Geometry: final body of the model. Coordinates: model frame, mm. A direction names the side the tool comes from. Coordinates: 2 decimals unless noted, no trailing zeros. Order: outer loops, then holes, each group sorted by start corner. A loop starts at its lowest first (then second) coordinate and runs counter-clockwise, first axis right, second up. Notation, with made-up numbers: M 37.5,-14 L 55.5,-14 A11 ccw 55.5,3 Z; hole C -14.75,-17.5 d8. An arc over 180 degrees is marked long. Use CSV: the item, a comma, the result in double quotes. Start each with the question number.
1. Pull-direction query (Y, two-part tool) for faces 1 (the cylindrical face through (7.395, -1.494, 6.294)), 2 (the flat face through (0, -6, 0)), 3 (the cylindrical face through (7.4, 6.03, -2.24)); classes: pulls with the +Y half, pulls with the -Y half, needs draft (parallel to the pull), parting line crosses it, or undercut.
2. Material intervals for line 1 (Y direction, x = 5.5, z = 0); line 2 (Y direction, x = -2.5, z = 0); line 3 (Y direction, x = 8, z = 5.5), sorted ascending.
3. First-contact query: P1, Ø5, axis at x = 1.5, y = -2.5, coming from the -Z side; P2, Ø1.1, axis at y = 4.5, z = 4.5, coming from the -X side; P3, Ø1, axis at x = -1.5, y = -3, coming from the +Z side. Flat tips, straight axial feed; report the tip coordinate or a pass-through.
4. Section query A-A on x = -3. Return the cut outline in (y, z).
5. Set-up query: faces 4 (the flat face through (-10, -1, 0)), 5 (the flat face through (0, -3, -5)). Return all of +Z, -Z, +X, -X, +Y, -Y with unobstructed straight access to the full face (end or side cutting, diameter ignored); none if empty.
from build123d import *
from build123d.topology import SkipClean

# Parameters (mm, degrees)
BASPROSKE_W      = 15
BASPROSKE_H      = 7.5
TOOTHCUT_DEPTH   = 19.371173071
TEETHCUTS_COUNT  = 13
TEETHCUTS_ANGLE  = 332.307692308
HUBNEAONESKE_R   = 5.249
HUBNEARONE_DEPTH = 10.0000508
BORSKE_R         = 0.4
BORE_DEPTH       = 25.0000508


with BuildPart() as part:
    # BasProSke → Base-Revolve (revolve)
    with BuildSketch(Plane(origin=(0, 0, 0), x_dir=(1, 0, 0), z_dir=(0, 1, 0)), mode=Mode.PRIVATE) as base_revolve_sk:
        with Locations((7.5, 3.75)):
            Rectangle(BASPROSKE_W, BASPROSKE_H)
    revolve(base_revolve_sk.sketch.rotate(Axis((-10, 0, 0), (1, 0, 0)), 180), axis=Axis((-10, 0, 0), (1, 0, 0)))

    # TooCutSke → ToothCut (cut, through all)
    with BuildSketch(Plane(origin=(0, 0, 0), x_dir=(0, 0, -1), z_dir=(1, 0, 0))):
        with BuildLine():
            ThreePointArc((0.550489643, 5.220053846), (0, 5.249), (-0.550489643, 5.220053846))
            ThreePointArc((-0.550489643, 5.220053846), (-0.834571714, 6.414617604), (-1.635166801, 7.345602405))
            ThreePointArc((-1.635166801, 7.345602405), (0, 7.5254), (1.635166801, 7.345602405))
            ThreePointArc((1.635166801, 7.345602405), (0.834571714, 6.414617604), (0.550489643, 5.220053846))
        make_face()
    toothcut = extrude(amount=TOOTHCUT_DEPTH, mode=Mode.SUBTRACT)

    # TeethCuts: ToothCut ×13 about axis
    teethcuts_axis = Axis((-10, 0, 0), (1, 0, 0))
    for i in range(1, TEETHCUTS_COUNT):
        add(toothcut.rotate(teethcuts_axis, i * TEETHCUTS_ANGLE / (TEETHCUTS_COUNT - 1)), mode=Mode.SUBTRACT)

    # HubNeaOneSke → HubNearOne (add)
    with SkipClean():  # the faces are left unmerged after this step: merging them gives an invalid solid
        with BuildSketch(Plane.ZY):
            Circle(HUBNEAONESKE_R)
        extrude(amount=HUBNEARONE_DEPTH)

    # BorSke → Bore (cut, symmetric)
    with SkipClean():  # the faces are left unmerged after this step: merging them gives an invalid solid
        with BuildSketch(Plane(origin=(0, 0, 0), x_dir=(0, 0, -1), z_dir=(1, 0, 0))):
            with Locations(Location((0, 0, 0), (0, 0, 180))):
                Circle(BORSKE_R)
        extrude(amount=BORE_DEPTH, both=True, mode=Mode.SUBTRACT)


solid = part.part
Results list:
1,face 1,"undercut"
1,face 2,"needs draft"
1,face 3,"undercut"
2,line 1,"y = -7.5 to -0.4, 0.4 to 5.25"
2,line 2,"y = -5.25 to -0.4, 0.4 to 5.25"
2,line 3,"y = -4.41 to -2.86, -1.46 to 0.1, 1.25 to 2.91"
3,P1,"stops at z = -7.47"
3,P2,"stops at x = 0"
3,P3,"stops at z = 4.62"
4,outline,"C 0,0 d10.5; hole C 0,0 d0.8"
5,face 4,"+Z, -Z, -X, +Y, -Y"
5,face 5,"-Z, -X, -Y"
